from build123d import *

# Parameters (mm, degrees)
SKETCH1_W                    = 7.62
SKETCH1_H                    = 1.5875
F_36_0_1065_DIAMETER_HOLE1_D = 2.7051
SCREW_PASSTHROUGHS_COUNT     = 12


with BuildPart() as part:
    # Sketch1 → Main (revolve)
    with BuildSketch(Plane.XY):
        with Locations((-41.91, 0.79375)):
            Rectangle(SKETCH1_W, SKETCH1_H)
    revolve(axis=Axis((0, 55, 0), (0, -1, 0)))

    # #36 (0.1065) Diameter Hole1 (through all)
    with Locations(Plane(origin=(0, 0, 0), x_dir=(-1, 0, 0), z_dir=(0, -1, 0))):
        with Locations((42.700575, 0)):
            f_36_0_1065_diameter_hole1 = Hole(F_36_0_1065_DIAMETER_HOLE1_D / 2)

    # Screw Passthroughs: #36 (0.1065) Diameter Hole1 ×12 about axis
    screw_passthroughs_axis = Axis((0, 0, 0), (0, 1, 0))
    for i in range(1, SCREW_PASSTHROUGHS_COUNT):
        add(f_36_0_1065_diameter_hole1.rotate(screw_passthroughs_axis, i * 360 / SCREW_PASSTHROUGHS_COUNT), mode=Mode.SUBTRACT)


solid = part.part
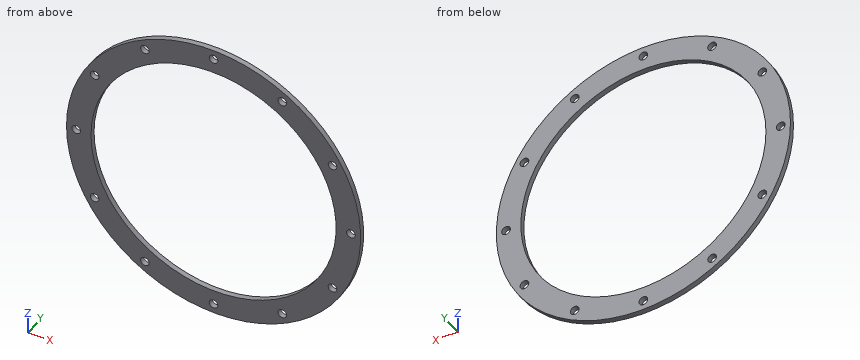
The model under review builds one solid part; all positions refer to its coordinate system, in mm. Give positions to 0.01 mm unless a question says otherwise; leave off trailing zeros. Order: outer loops, then holes, each group sorted by start corner. A loop starts at its lowest first (then second) coordinate and runs counter-clockwise, first axis right, second up. Notation, with made-up numbers: M 24,-32 L 29,-32 A33 ccw 29,6 Z; hole C 5.25,27 d11. An arc over 180 degrees is marked long. Answer in a Markdown table with one row per item. Add a question column.
1. Add section B-B on z = 0. State the section outline as (x, y) points.
2. Add section A-A on x = 0. State the section outline as (y, z) points, plus the area to 3 significant figures.
3. Add section D-D on x = -29. State the section outline as (y, z) points, plus the area to 3 significant figures.
4. Add section C-C on z = 28.5. State the section outline as (x, y) points, plus the area to 3 significant figures.
5. To check wall thickness, follow line 1 along X through (y, z) = (1.35, -9.5); line 2 along Z through (x, y) = (24, 1); line 3 along X through (y, z) = (0.75, 31). State the ranges of each line that lie inside material, in increasing order.
The answers:
| question | item | result |
|---|---|---|
| 1 | outline | M -45.72,0 L -44.05,0 L -44.05,1.59 L -45.72,1.59 Z; M -41.35,0 L -38.1,0 L -38.1,1.59 L -41.35,1.59 Z; M 38.1,0 L 41.35,0 L 41.35,1.59 L 38.1,1.59 Z; M 44.05,0 L 45.72,0 L 45.72,1.59 L 44.05,1.59 Z |
| 2 | outline | M 0,-45.72 L 1.59,-45.72 L 1.59,-44.05 L 0,-44.05 Z; M 0,-41.35 L 1.59,-41.35 L 1.59,-38.1 L 0,-38.1 Z; M 0,38.1 L 1.59,38.1 L 1.59,41.35 L 0,41.35 Z; M 0,44.05 L 1.59,44.05 L 1.59,45.72 L 0,45.72 Z |
| 2 | area | 15.6 mm2 |
| 3 | outline | M 0,-35.35 L 1.59,-35.35 L 1.59,-24.71 L 0,-24.71 Z; M 0,24.71 L 1.59,24.71 L 1.59,35.35 L 0,35.35 Z |
| 3 | area | 33.8 mm2 |
| 4 | outline | M -35.75,0 L -25.29,0 L -25.29,1.59 L -35.75,1.59 Z; M 25.29,0 L 35.75,0 L 35.75,1.59 L 25.29,1.59 Z |
| 4 | area | 33.2 mm2 |
| 5 | line 1 | -44.72 to -36.9, 36.9 to 44.72 |
| 5 | line 2 | -38.91 to -29.59, 29.59 to 38.91 |
| 5 | line 3 | -33.61 to -22.15, 22.15 to 33.61 |
